Work out the finished part from the listing and answer in its coordinate system (mm). A direction names the side the tool comes from. Round coordinates to 2 decimals unless told otherwise and drop trailing zeros. Order: outer loops, then holes, each group sorted by start corner. A loop starts at its lowest first (then second) coordinate and runs counter-clockwise, first axis right, second up. Notation, with made-up numbers: M 70,45 L 120,45 A26 ccw 120,63 Z; hole C 52.25,-5 d10. An arc over 180 degrees is marked long. Return JSON: item names as keys, results as strings.
from build123d import *

# Parameters (mm, degrees)
SKETCH1_W             = 85.598
SKETCH1_H             = 53.34
BOSS_EXTRUDE1_DEPTH   = 2.159
SKETCH2_W             = 85.598
SKETCH2_H             = 2.159
BOSS_EXTRUDE2_DEPTH   = 9.271
FILLET1_R             = 1.27
FILLET2_R             = 1.27
FILLET3_R             = 2.54
SKETCH3_W             = 29.21
SKETCH3_H             = 33.02
CUT_EXTRUDE1_DEPTH    = 52.273723699
FILLET5_R             = 5.08
F_4_CLEARANCE_HOLE1_D = 3.2639
SKETCH18_R            = 3.81
BOSS_EXTRUDE6_DEPTH   = 3.048
SKETCH19_R            = 1.9685
CUT_EXTRUDE7_DEPTH    = 3.429
SKETCH20_R            = 0.9525
CUT_EXTRUDE8_DEPTH    = 52.343981195
CUT_EXTRUDE9_DEPTH    = 52.273723699
FILLET6_R             = 2.54
FILLET7_R             = 7.62
CUT_EXTRUDE10_DEPTH   = 52.273723699
FILLET8_R             = 2.54
FILLET9_R             = 7.62


with BuildPart() as part:
    # Sketch1 → Boss-Extrude1 (new body)
    with BuildSketch(Plane.XY):
        Rectangle(SKETCH1_W, SKETCH1_H)
    extrude(amount=BOSS_EXTRUDE1_DEPTH)

    # Sketch2 → Boss-Extrude2 (add)
    with BuildSketch(Plane.XY.offset(2.159)):
        with Locations((0, 25.5905)):
            Rectangle(SKETCH2_W, SKETCH2_H)
    extrude(amount=BOSS_EXTRUDE2_DEPTH)

    # Fillet1
    fillet1_edges = [part.edges().sort_by_distance(p)[0] for p in [
        (0, 24.511, 2.159),
    ]]
    fillet(fillet1_edges, radius=FILLET1_R)

    # Fillet2
    fillet2_edges = [part.edges().sort_by_distance(p)[0] for p in [
        (0, 26.67, 0),
    ]]
    fillet(fillet2_edges, radius=FILLET2_R)

    # Fillet3
    fillet3_edges = [part.edges().sort_by_distance(p)[0] for p in [
        (42.799, 25.5905, 11.43),
        (-42.799, 25.5905, 11.43),
    ]]
    fillet(fillet3_edges, radius=FILLET3_R)

    # Sketch3 → Cut-Extrude1 (cut, through all)
    with BuildSketch(Plane.XY.offset(2.159)):
        with Locations((0, -3.81)):
            Rectangle(SKETCH3_W, SKETCH3_H)
    extrude(amount=-CUT_EXTRUDE1_DEPTH, mode=Mode.SUBTRACT)

    # Fillet5
    fillet5_edges = [part.edges().sort_by_distance(p)[0] for p in [
        (-14.605, -20.32, 1.0795),
        (-14.605, 12.7, 1.0795),
        (14.605, 12.7, 1.0795),
        (14.605, -20.32, 1.0795),
    ]]
    fillet(fillet5_edges, radius=FILLET5_R)

    # #4 Clearance Hole1 (through all)
    with Locations(Plane(origin=(0, 24.511, 0), x_dir=(-1, 0, 0), z_dir=(0, -1, 0))):
        with Locations((-38.1, -7.62), (24.13, -7.62)):
            Hole(F_4_CLEARANCE_HOLE1_D / 2)

    # Sketch18 → Boss-Extrude6 (add)
    with BuildSketch(Plane.XY.offset(2.159)):
        with Locations(Location((-23.18312986, -1.143, 0), (0, 0, 180))):
            Circle(SKETCH18_R)
        with Locations(Location((-23.18312986, -18.923, 0), (0, 0, 180))):
            Circle(SKETCH18_R)
        with Locations(Location((21.77487014, -10.033, 0), (0, 0, 180))):
            Circle(SKETCH18_R)
    extrude(amount=BOSS_EXTRUDE6_DEPTH)

    # Sketch19 → Cut-Extrude7 (cut)
    with BuildSketch(Plane.XY.offset(5.207)):
        with Locations((-23.18312986, -18.923)):
            Circle(SKETCH19_R)
        with Locations((21.77487014, -10.033)):
            Circle(SKETCH19_R)
        with Locations((-23.18312986, -1.143)):
            Circle(SKETCH19_R)
    extrude(amount=-CUT_EXTRUDE7_DEPTH, mode=Mode.SUBTRACT)

    # Sketch20 → Cut-Extrude8 (cut, through all)
    with BuildSketch(Plane.XY.offset(1.778)):
        with Locations((-23.18312986, -1.143)):
            Circle(SKETCH20_R)
        with Locations((-23.18312986, -18.923)):
            Circle(SKETCH20_R)
        with Locations((21.77487014, -10.033)):
            Circle(SKETCH20_R)
    extrude(amount=-CUT_EXTRUDE8_DEPTH, mode=Mode.SUBTRACT)

    # Sketch21 → Cut-Extrude9 (cut, through all)
    with BuildSketch(Plane.XY.offset(2.159)):
        with BuildLine():
            Line((-42.799, 12.7), (-37.719, 12.7))
            ThreePointArc((-37.719, 12.7), (-34.126897552, 11.212102448), (-32.639, 7.62))
            Line((-32.639, 7.62), (-32.639, -26.67))
            Line((-32.639, -26.67), (-42.799, -26.67))
            Line((-42.799, -26.67), (-42.799, 12.7))
        make_face()
    extrude(amount=-CUT_EXTRUDE9_DEPTH, mode=Mode.SUBTRACT)

    # Fillet6
    fillet6_edges = [part.edges().sort_by_distance(p)[0] for p in [
        (-42.799, 12.7, 1.0795),
    ]]
    fillet(fillet6_edges, radius=FILLET6_R)

    # Fillet7
    fillet7_edges = [part.edges().sort_by_distance(p)[0] for p in [
        (-32.639, -26.67, 1.0795),
    ]]
    fillet(fillet7_edges, radius=FILLET7_R)

    # Sketch22 → Cut-Extrude10 (cut, through all)
    with BuildSketch(Plane.XY.offset(2.159)):
        with BuildLine():
            Line((42.799, 12.7), (42.037, 12.7))
            ThreePointArc((42.037, 12.7), (38.444897552, 11.212102448), (36.957, 7.62))
            Line((36.957, 7.62), (36.957, -26.67))
            Line((36.957, -26.67), (42.799, -26.67))
            Line((42.799, -26.67), (42.799, 12.7))
        make_face()
    extrude(amount=-CUT_EXTRUDE10_DEPTH, mode=Mode.SUBTRACT)

    # Fillet8
    fillet8_edges = [part.edges().sort_by_distance(p)[0] for p in [
        (42.799, 12.7, 1.0795),
    ]]
    fillet(fillet8_edges, radius=FILLET8_R)

    # Fillet9
    fillet9_edges = [part.edges().sort_by_distance(p)[0] for p in [
        (36.957, -26.67, 1.0795),
    ]]
    fillet(fillet9_edges, radius=FILLET9_R)


solid = part.part
Item 1: Find section D-D (x = 38.1). Determine the outline of the cut face in (y, z), plus the area to 3 significant figures.
Output:
{"outline": "M 10.83,0 L 25.4,0 A1.27 ccw 26.67,1.27 L 26.67,5.99 L 24.51,5.99 L 24.51,3.43 A1.27 cw 23.24,2.16 L 10.83,2.16 Z; M 24.51,9.25 L 26.67,9.25 L 26.67,11.43 L 24.51,11.43 Z", "area": "47.2 mm^2"}
Item 2: Find section A-A (x = -1). Determine the outline of the cut face in (y, z), plus the area to 3 significant figures.
Output:
{"outline": "M -26.67,0 L -20.32,0 L -20.32,2.16 L -26.67,2.16 Z; M 12.7,0 L 25.4,0 A1.27 ccw 26.67,1.27 L 26.67,11.43 L 24.51,11.43 L 24.51,3.43 A1.27 cw 23.24,2.16 L 12.7,2.16 Z", "area": "63.9 mm^2"}
Item 3: Which of the six approach directions +Z, -Z, +X, -X, +Y, -Y give full straight-line access (tool end or side, diameter ignored) to faces 5 (the flat face through (36.957, -6, 1)), 6 (the flat face through (0, 12.7, 1)), 7 (the cylindrical face through (21.52, -8.08, 3.52))?
Output:
{"face 5": "+Z, -Z, +X, -Y", "face 6": "+Z, -Z", "face 7": "+Z"}
Item 4: Find section C-C (y = 9). Determine the outline of the cut face in (x, z).
Output:
{"outline": "M -32.83,0 L -14.41,0 L -14.41,2.16 L -32.83,2.16 Z; M 14.41,0 L 37.15,0 L 37.15,2.16 L 14.41,2.16 Z"}
Item 5: Find section B-B (z = 7.62). Determine the outline of the cut face in (x, y), plus the area to 3 significant figures.
Output:
{"outline": "M -42.8,24.51 L -25.76,24.51 L -25.76,26.67 L -42.8,26.67 Z; M -22.5,24.51 L 36.47,24.51 L 36.47,26.67 L -22.5,26.67 Z; M 39.73,24.51 L 42.8,24.51 L 42.8,26.67 L 39.73,26.67 Z", "area": "171 mm^2"}
Item 6: Consider line 1 along X through (y, z) = (26.05, 7.62); line 2 along Z through (x, y) = (-24, 25); line 3 along X through (y, z) = (-5.5, 1.75) (3 decimals). Determine where each line is inside the solid, lowest interval first. Write a range as [from, to].
Output:
{"line 1": "x = [-42.8, -25.76], [-22.5, 36.47], [39.73, 42.8]", "line 2": "z = [0, 5.99], [9.25, 11.43]", "line 3": "x = [-32.639, -14.605], [14.605, 36.957]"}
Item 7: Each of these flat-tipped pins is pushed along its axis until it touches: pin 1 (2 mm diameter, centred on x = 22, y = -9, fed in from +Z); pin 2 (12 mm diameter, centred on x = 11, y = -13, fed in from +Z); pin 3 (1.1 mm diameter, centred on y = -2, z = 1.5, fed in from +X); pin 4 (1 mm diameter, centred on x = 14, y = -3, fed in from +Z). Where does it stop, or does it pass through?
Output:
{"pin 1": "stops at z = 5.21", "pin 2": "stops at z = 2.16", "pin 3": "stops at x = 36.96", "pin 4": "passes through"}
Item 8: The mould has two halves that part along X. Classify faces 1 (the flat face through (-1, 15, 2.159)), 2 (the cylindrical face through (-24.94, -15.54, 3.66)), 3 (the cylindrical face through (-22.125, -17.263, 3.517)), 4 (the flat face through (42.799, 23, 1)): pulls with the +X half, pulls with the -X half, needs draft (parallel to the pull), parting line crosses it, or undercut.
Output:
{"face 1": "needs draft", "face 2": "parting line crosses it", "face 3": "undercut", "face 4": "pulls with the +X half"}
